Work out the finished part from the listing and answer in its coordinate system (mm). Face numbers are marked on the shaded views. A direction names the side the tool comes from. Round coordinates to 2 decimals unless told otherwise and drop trailing zeros. Write each loop counter-clockwise with the first axis right and the second up, starting at its lowest first coordinate (ties: lowest second). Pieces come first, ordered by that corner, then holes. Notation, with made-up numbers: M 7.5,0.25 L 40.5,0.25 A23 cw 40.5,21.25 Z; hole C -22,72 d1. An arc over 180 degrees is marked long. Answer in a Markdown table with one row per item.
```python
from build123d import *

# Parameters (mm, degrees)
F1_DEPTH = 25.4
F2_R     = 6.35
F3_DEPTH = 25.4
F4_R     = 0.79375
F6_DEPTH = 25.4
F5_R     = 0.79375
F7_DEPTH = 25.4


with BuildPart() as f1:
    # F0 (on Front) → F1 (new body)
    with BuildSketch(Plane.XZ):
        Polygon((-13.930467, 28.698625), (-13.930467, -3.051375), (-10.755467, -3.051375), (-10.755467, 25.523625), (33.694533, 25.523625), (33.694533, -3.051375), (36.869533, -3.051375), (36.869533, 28.698625), align=None)
    extrude(amount=F1_DEPTH)

    # F2 (on face) → F3 (cut)
    with BuildSketch(Plane.XY.offset(28.698625)):
        with Locations((11.469533, -12.7)):
            Circle(F2_R)
    extrude(amount=-F3_DEPTH, mode=Mode.SUBTRACT)

    # F4 (on face) → F6 (cut)
    with BuildSketch(Plane(origin=(0, 0, -3.051375), x_dir=(1, 0, 0), z_dir=(0, 0, -1))):
        with Locations((-12.342967, 19.05)):
            Circle(F4_R)
        with Locations((-12.342967, 6.35)):
            Circle(F4_R)
    extrude(amount=-F6_DEPTH, mode=Mode.SUBTRACT)

    # F5 (on face) → F7 (cut)
    with BuildSketch(Plane(origin=(0, 0, -3.051375), x_dir=(1, 0, 0), z_dir=(0, 0, -1))):
        with Locations((35.269333, 19.05)):
            Circle(F5_R)
        with Locations((35.269333, 6.349987)):
            Circle(F5_R)
    extrude(amount=-F7_DEPTH, mode=Mode.SUBTRACT)


solid = f1.part
```
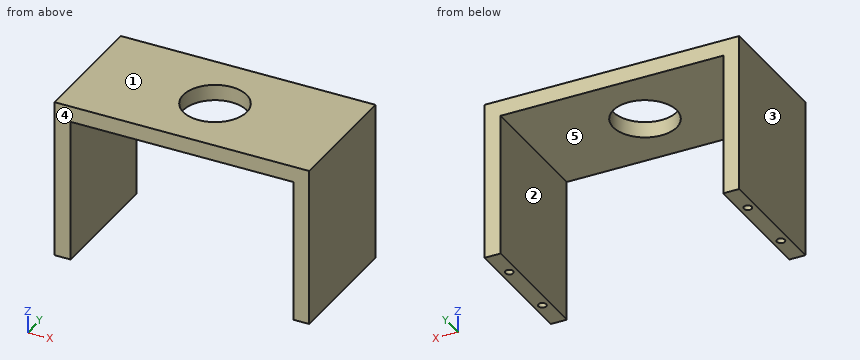
1. The part is cut by section D-D (y = -22.25). Determine the outline of the cut face in (x, z), plus the area to 3 significant figures.
Calculated:
| item | result |
|---|---|
| outline | M -13.93,-3.05 L -10.76,-3.05 L -10.76,25.52 L 33.69,25.52 L 33.69,-3.05 L 36.87,-3.05 L 36.87,28.7 L -13.93,28.7 Z |
| area | 343 mm² |
2. A tool of negligible diameter and unlimited length cuts with its end or side. For the marked faces 1 and 2, from which of +Z, -Z, +X, -X, +Y, -Y can it reach the whole face along a straight path? Write none if from no direction.
Calculated:
| item | result |
|---|---|
| face 1 | +Z, +X, -X, +Y, -Y |
| face 2 | -Z, +Y, -Y |
3. The part is cut by section A-A (y = -12.7). Determine the outline of the cut face in (x, z).
Calculated:
| item | result |
|---|---|
| outline | M -13.93,-3.05 L -10.76,-3.05 L -10.76,25.52 L 5.12,25.52 L 5.12,28.7 L -13.93,28.7 Z; M 17.82,25.52 L 33.69,25.52 L 33.69,-3.05 L 36.87,-3.05 L 36.87,28.7 L 17.82,28.7 Z |
4. The part is cut by section C-C (x = 11). Determine the outline of the cut face in (y, z), plus the area to 3 significant figures.
Calculated:
| item | result |
|---|---|
| outline | M -25.4,25.52 L -19.03,25.52 L -19.03,28.7 L -25.4,28.7 Z; M -6.37,25.52 L 0,25.52 L 0,28.7 L -6.37,28.7 Z |
| area | 40.4 mm² |
5. Consider line 1 along X through (y, z) = (-19.05, 12.75); line 2 along X through (y, z) = (-23.25, 0.5); line 3 along Z through (x, y) = (4.5, -7.5). Determine where each line is inside the solid, lowest interval first. Write a range as from..to.
Calculated:
| item | result |
|---|---|
| line 1 | x = -13.93..-13.14, -11.55..-10.76, 33.69..34.48, 36.06..36.87 |
| line 2 | x = -13.93..-10.76, 33.69..36.87 |
| line 3 | z = 25.52..28.7 |
6. Determine the mould class of the marked faces 3, 4 and 5 for opening direction X: released by +X, released by -X, zero draft, split by the parting line, or undercut.
Calculated:
| item | result |
|---|---|
| face 3 | released by -X |
| face 4 | zero draft |
| face 5 | undercut |
7. Given pin 1 (1.7 mm diameter, centred on x = -12.5, y = -6, fed in from -Z); pin 2 (12 mm diameter, centred on x = 23.5, z = 9, fed in from +Y); pin 3 (0.8 mm diameter, centred on x = 35, y = -19, fed in from -Z), each flat-ended and moving along its own axis, determine where each tip first touches the part or whether it passes through.
Calculated:
| item | result |
|---|---|
| pin 1 | stops at z = -3.05 |
| pin 2 | passes through |
| pin 3 | stops at z = 22.35 |
8. The part is cut by section B-B (z = 24.5). Determine the outline of the cut face in (x, y), plus the area to 3 significant figures.
Calculated:
| item | result |
|---|---|
| outline | M -13.93,-25.4 L -10.76,-25.4 L -10.76,0 L -13.93,0 Z; M 33.69,-25.4 L 36.87,-25.4 L 36.87,0 L 33.69,0 Z |
| area | 161 mm² |
